Could you check a few things on this drawing? It's one solid part, dimensions in mm from its lowest x, y, z. Coordinates: 2 decimals unless noted, no trailing zeros. Order: outer loops, then holes, each group sorted by start corner. A loop starts at its lowest first (then second) coordinate and runs counter-clockwise, first axis right, second up. Notation, with made-up numbers: (52, -31) -> (81, -31) arc R11 cw to (81, -24) -> close; hole circle Ø5 at (33, 29.25). An arc over 180 degrees is marked (long way). Use a Markdown table: item, result. Add a question column.
1. Suppose I cut it at A-A, the plane x = 38. List the corners of the cut face in (y, z) for me.
2. Suppose I cut it at D-D, the plane x = 15. List the corners of the cut face in (y, z) for me.
3. Suppose I cut it at C-C, the plane z = 1.85. List the corners of the cut face in (x, y) for me, then the cut area to 3 significant figures.
4. If I drill on line 1 along Y through (x, z) = (38, 1.7); line 2 along Y through (x, z) = (15, 2.3); line 3 along X through (y, z) = (46.5, 0.85), over which ranges is the centre line in solid material (lowest first)? Write a range as from..to.
5. Suppose I cut it at B-B, the plane y = 49. List the corners of the cut face in (x, z) for me, then the cut area to 3 significant figures.
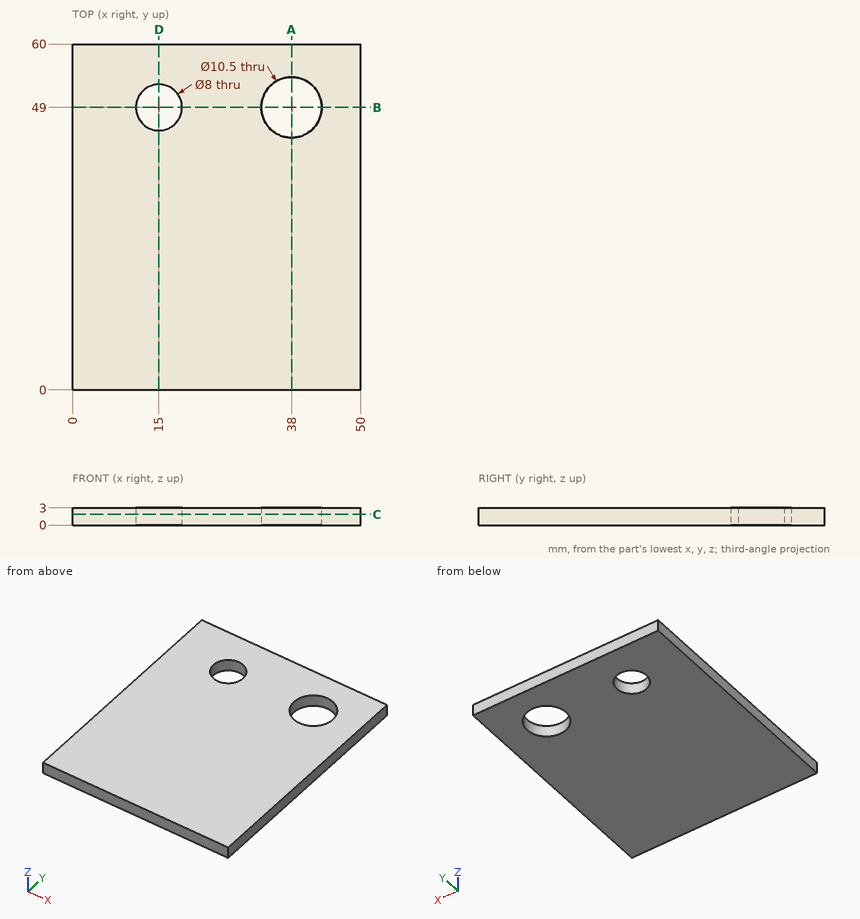
Worked out:
| question | item | result |
|---|---|---|
| 1 | outline | (0, 0) -> (43.75, 0) -> (43.75, 3) -> (0, 3) -> close; (54.25, 0) -> (60, 0) -> (60, 3) -> (54.25, 3) -> close |
| 2 | outline | (0, 0) -> (45, 0) -> (45, 3) -> (0, 3) -> close; (53, 0) -> (60, 0) -> (60, 3) -> (53, 3) -> close |
| 3 | outline | (0, 0) -> (50, 0) -> (50, 60) -> (0, 60) -> close; hole circle Ø8 at (15, 49); hole circle Ø10.5 at (38, 49) |
| 3 | area | 2,860 mm² |
| 4 | line 1 | y = 0..43.75, 54.25..60 |
| 4 | line 2 | y = 0..45, 53..60 |
| 4 | line 3 | x = 0..11.88, 18.12..33.38, 42.62..50 |
| 5 | outline | (0, 0) -> (11, 0) -> (11, 3) -> (0, 3) -> close; (19, 0) -> (32.75, 0) -> (32.75, 3) -> (19, 3) -> close; (43.25, 0) -> (50, 0) -> (50, 3) -> (43.25, 3) -> close |
| 5 | area | 94.5 mm² |
